Input: part model. Units: mm. Frame: model coordinates. Coordinates: 2 decimals unless noted, no trailing zeros. Loops run counter-clockwise (first coordinate to the right, second up) from the corner with the lowest first, then second, coordinate; pieces in that order, holes last. Notation, with made-up numbers: (52.25, 56.25) -> (111.25, 56.25) arc R20 ccw to (111.25, 84.25) -> close; hole circle Ø6 at (-9, -27.5). An arc over 180 degrees is marked (long way). Put each result on its own line as item: value. Start each with the question number.
1) Contact query for flat-ended pins moving along their axis: P1, Ø2.5, axis at x = -24.5, z = 29, coming from the -Y side; P2, Ø3.5, axis at x = 24.5, z = -29, coming from the -Y side. Output: stop coordinate, or through.
2) Material intervals for L1, parallel to X at y = 1.4, z = 29; L2, parallel to X at y = 1.4, z = -35; L3, parallel to Z at x = -15, y = 0.6, sorted ascending.
3) Cut plane A-A (x = -24.5). Return the cut outline in (y, z), plus the area to 3 significant figures.
4) Cut plane B-B (z = -23). Return the cut outline in (x, y), plus the area to 3 significant figures.
5) Cut plane D-D (x = 6.5). Return the cut outline in (y, z).
6) Cut plane C-C (y = 1.1). State how many separate pieces and enclosed holes the cut face has, plus the area to 3 significant figures.
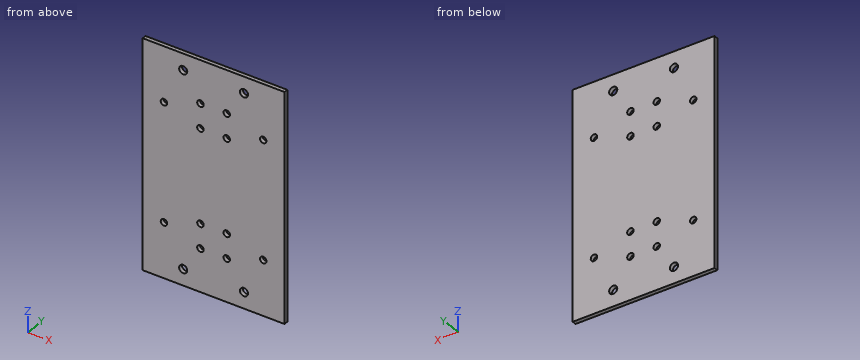
from build123d import *

# Parameters (mm, degrees)
SKETCH_2_W          = 70
SKETCH_2_H          = 112
SKETCH_2_R          = 1.6
EXTRUDE_1_DEPTH     = 2
SKETCH_3_R          = 2
CUT_EXTRUDE_1_DEPTH = 3


with BuildPart() as part:
    # 草圖2 → 填料-伸長1 (new body)
    with BuildSketch(Plane(origin=(0, 0, 0), x_dir=(1, 0, 0), z_dir=(0, 1, 0))):
        Rectangle(SKETCH_2_W, SKETCH_2_H)
        with Locations((-6.5, 35)):
            Circle(SKETCH_2_R, mode=Mode.SUBTRACT)
        with Locations((-6.5, -35)):
            Circle(SKETCH_2_R, mode=Mode.SUBTRACT)
        with Locations((-6.5, 23)):
            Circle(SKETCH_2_R, mode=Mode.SUBTRACT)
        with Locations((-6.5, -23)):
            Circle(SKETCH_2_R, mode=Mode.SUBTRACT)
        with Locations((6.5, -35)):
            Circle(SKETCH_2_R, mode=Mode.SUBTRACT)
        with Locations((6.5, -23)):
            Circle(SKETCH_2_R, mode=Mode.SUBTRACT)
        with Locations((6.5, 23)):
            Circle(SKETCH_2_R, mode=Mode.SUBTRACT)
        with Locations((6.5, 35)):
            Circle(SKETCH_2_R, mode=Mode.SUBTRACT)
        with Locations((-24.5, 29)):
            Circle(SKETCH_2_R, mode=Mode.SUBTRACT)
        with Locations((24.5, 29)):
            Circle(SKETCH_2_R, mode=Mode.SUBTRACT)
        with Locations((-24.5, -29)):
            Circle(SKETCH_2_R, mode=Mode.SUBTRACT)
        with Locations((24.5, -29)):
            Circle(SKETCH_2_R, mode=Mode.SUBTRACT)
    extrude(amount=EXTRUDE_1_DEPTH)

    # 草圖3 → 除料-伸長1 (cut, through all)
    with BuildSketch(Plane(origin=(0, 2, 0), x_dir=(1, 0, 0), z_dir=(0, 1, 0))):
        with Locations((-15, -48)):
            Circle(SKETCH_3_R)
        with Locations((-15, 48)):
            Circle(SKETCH_3_R)
        with Locations((15, -48)):
            Circle(SKETCH_3_R)
        with Locations((15, 48)):
            Circle(SKETCH_3_R)
    extrude(amount=-CUT_EXTRUDE_1_DEPTH, mode=Mode.SUBTRACT)


solid = part.part
Results found:
1. P1: passes through
1. P2: stops at y = 0
2. L1: x = -35 to -26.1, -22.9 to 22.9, 26.1 to 35
2. L2: x = -35 to -8.1, -4.9 to 4.9, 8.1 to 35
2. L3: z = -56 to -50, -46 to 46, 50 to 56
3. outline: (0, -56) -> (2, -56) -> (2, -30.6) -> (0, -30.6) -> close; (0, -27.4) -> (2, -27.4) -> (2, 27.4) -> (0, 27.4) -> close; (0, 30.6) -> (2, 30.6) -> (2, 56) -> (0, 56) -> close
3. area: 211 mm2
4. outline: (-35, 0) -> (-8.1, 0) -> (-8.1, 2) -> (-35, 2) -> close; (-4.9, 0) -> (4.9, 0) -> (4.9, 2) -> (-4.9, 2) -> close; (8.1, 0) -> (35, 0) -> (35, 2) -> (8.1, 2) -> close
4. area: 127 mm2
5. outline: (0, -56) -> (2, -56) -> (2, -36.6) -> (0, -36.6) -> close; (0, -33.4) -> (2, -33.4) -> (2, -24.6) -> (0, -24.6) -> close; (0, -21.4) -> (2, -21.4) -> (2, 21.4) -> (0, 21.4) -> close; (0, 24.6) -> (2, 24.6) -> (2, 33.4) -> (0, 33.4) -> close; (0, 36.6) -> (2, 36.6) -> (2, 56) -> (0, 56) -> close
6. separate pieces: 1
6. enclosed holes: 16
6. area: 7,690 mm2
